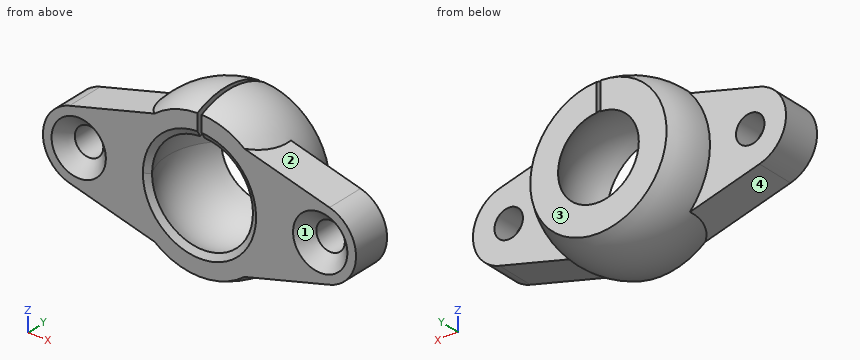
from build123d import *

# Parameters (mm, degrees)
ESQUISSE3_R                          = 1.65
BOSS_EXTRU_1_DEPTH                   = 4.5
CHANFREIN1_SIZE                      = 1.5
ENL_V_DE_MAT_EXTRU_MINCE1_DEPTH      = 23.312440476
ENL_V_DE_MAT_EXTRU_MINCE1_DEPTH_BACK = 23.312440476
ESQUISSE4_W                          = 0.5
ESQUISSE4_H                          = 9.35


with BuildPart() as part:
    # Esquisse1 → Révolution1 (revolve)
    with BuildSketch(Plane.XY):
        with BuildLine():
            Line((-5.85, -3.563705936), (-6.566198339, -4))
            Line((-6.566198339, -4), (-8.451183349, -4))
            ThreePointArc((-8.451183349, -4), (-9.332564872, 0.570730153), (-7.9007911, 5))
            Line((-7.9007911, 5), (-4.682146943, 5))
            ThreePointArc((-4.682146943, 5), (-6.787178696, 0.925583789), (-5.85, -3.563705936))
        make_face()
    revolve(axis=Axis((0, 11.493598295, 0), (0, -1, 0)))

    # Esquisse3 → Boss.-Extru.1 (add)
    # profile 1 of 2: a face of its own
    with BuildSketch(Plane.XZ.offset(4)):
        with BuildLine():
            Line((-15.074099037, 4.008592179), (-3.376482998, 7.14295895))
            ThreePointArc((-3.376482998, 7.14295895), (-7.9007911, 0), (-3.376482998, -7.14295895))
            Line((-3.376482998, -7.14295895), (-15.074099037, -4.008592179))
            ThreePointArc((-15.074099037, -4.008592179), (-18.15, 0), (-15.074099037, 4.008592179))
        make_face()
        with Locations((-14, 0)):
            Circle(ESQUISSE3_R, mode=Mode.SUBTRACT)
    # profile 2 of 2: a face of its own
    with BuildSketch(Plane.XZ.offset(4)):
        with BuildLine():
            Line((15.074099037, 4.008592179), (3.376482998, 7.14295895))
            ThreePointArc((3.376482998, 7.14295895), (7.9007911, 0), (3.376482998, -7.14295895))
            Line((3.376482998, -7.14295895), (15.074099037, -4.008592179))
            ThreePointArc((15.074099037, -4.008592179), (18.15, 0), (15.074099037, 4.008592179))
        make_face()
        with Locations((14, 0)):
            Circle(ESQUISSE3_R, mode=Mode.SUBTRACT)
    extrude(amount=-BOSS_EXTRU_1_DEPTH)

    # Chanfrein1
    chanfrein1_edges = [part.edges().sort_by_distance(p)[0] for p in [
        (12.35, -4, 0),
        (-15.65, -4, 0),
    ]]
    chamfer(chanfrein1_edges, length=CHANFREIN1_SIZE)

    # Esquisse4 → Enlèv. de mat.-Extru.-Mince1 (cut, two sides: drawn at the far end of the back side and taken through both)
    with BuildSketch(Plane(origin=(0, 5, 0), x_dir=(1, 0, 0), z_dir=(0, 1, 0)).offset(-ENL_V_DE_MAT_EXTRU_MINCE1_DEPTH_BACK)):
        with Locations((0, -4.675)):
            Rectangle(ESQUISSE4_W, ESQUISSE4_H)
    extrude(amount=ENL_V_DE_MAT_EXTRU_MINCE1_DEPTH + ENL_V_DE_MAT_EXTRU_MINCE1_DEPTH_BACK, mode=Mode.SUBTRACT)


solid = part.part
Here's how the part is built. I have some questions about the finished solid (model axes, mm). Face numbers are marked on the shaded views. Coordinates: 2 decimals unless noted, no trailing zeros. Write each loop counter-clockwise with the first axis right and the second up, starting at its lowest first coordinate (ties: lowest second). Pieces come first, ordered by that corner, then holes.
Item 1: If I drill on line 1 (X direction, y = -0.5, z = 0.75); line 2 (X direction, y = -3.25, z = 7); line 3 (X direction, y = 1.5, z = -2.75), over which ranges is the centre line in solid material (lowest first)?
Item 2: If we mould it in two halves opening along X, with no side actions, what happens to the marked faces 1, 2, 3 and 4? For each: +X half, -X half, draft (parallel to the pull), parting line (faces both ways), or undercut.
Item 3: Will these pins go through, and if not, where does the flat tip stop? pin 1 (5.5 mm diameter, centred on x = -13, z = -2, fed in from +Y); pin 2 (5 mm diameter, centred on x = 1, z = -1, fed in from +Y); pin 3 (1.5 mm diameter, centred on x = 3.5, y = 2, fed in from +Z); pin 4 (4 mm diameter, centred on y = 3, z = -1.5, fed in from -X).
Item 4: I want a section at B-B on y = -1. Write out the boundary of the cut face in (x, z).
Item 5: I want a section at D-D on y = 1.75. Write out the boundary of the cut face in (x, z), and give its area (3 significant figures).
Item 6: I want a section at C-C on x = -10. Write out the boundary of the cut face in (y, z).
Item 7: I want a section at A-A on x = 14. Write out the boundary of the cut face in (y, z).
Findings below:
1. line 1: x = -18.08 to -15.47, -12.53 to -6.79, 6.79 to 12.53, 15.47 to 18.08
1. line 2: x = -5.28 to -0.25, 0.25 to 5.28
1. line 3: x = -8.81 to -6.09, 6.09 to 8.81
2. face 1: undercut
2. face 2: +X half
2. face 3: draft
2. face 4: -X half
3. pin 1: stops at y = 0.5
3. pin 2: passes through
3. pin 3: stops at z = 8.76
3. pin 4: stops at x = -9.25
4. outline: (-15.07, -4.01) - (-6.94, -6.19) arc R9.3 ccw to (6.94, -6.19) - (15.07, -4.01) arc R4.15 ccw to (15.07, 4.01) - (6.94, 6.19) arc R9.3 ccw to (0.25, 9.29) - (0.25, 6.77) arc R6.78 cw (long way) to (-0.25, 6.77) - (-0.25, 9.29) arc R9.3 ccw to (-6.94, 6.19) - (-15.07, 4.01) arc R4.15 ccw to start; hole circle Ø3.3 at (-14, 0); hole circle Ø3.3 at (14, 0)
5. outline: (-0.25, 6.62) - (-0.25, 9.18) arc R9.18 ccw (long way) to (0.25, 9.18) - (0.25, 6.62) arc R6.62 cw (long way) to start
5. area: 126 mm2
6. outline: (-4, -5.37) - (0.5, -5.37) - (0.5, 5.37) - (-4, 5.37) - close
7. outline: (-4, -4.3) - (0.5, -4.3) - (0.5, -1.65) - (-2.5, -1.65) - (-4, -3.15) - close; (-4, 3.15) - (-2.5, 1.65) - (0.5, 1.65) - (0.5, 4.3) - (-4, 4.3) - close
